Source: CAD feature listing. Evaluate the final solid. Frame: model axes, mm. Coordinates: 2 decimals unless noted, no trailing zeros. Order: outer loops, then holes, each group sorted by start corner. A loop starts at its lowest first (then second) coordinate and runs counter-clockwise, first axis right, second up.
Item 1: Contact query for flat-ended pins moving along their axis: P1, Ø3.5, axis at x = 100, z = 130, coming from the +Y side; P2, Ø8, axis at x = -108, z = 30.32, coming from the -Y side. Output: stop coordinate, or through.
Item 2: Section B-B on z = -89.5. Return the cut outline in (x, y), then the cut area to 3 significant figures.
Item 3: Section C-C on z = -40.5. Return the cut outline in (x, y), then the cut area to 3 significant figures.
Item 4: Mould query, pull axis X, two halves, no side actions, for faces 1 (the flat face through (130, 3, 2)), 2 (the flat face through (-100, 3, 78)). Classes: released by +X, released by -X, zero draft, split by the parting line, or undercut.
Item 5: Ray query, line 1 (X direction, y = 4.75, z = 130); line 2 (Z direction, x = 39.5, y = 1); line 3 (Z direction, x = -108, y = 2.75). Return the intervals inside material, ascending.
Item 6: Section D-D on y = 1.5. State how many separate pieces and enclosed holes the cut face has, then the cut area to 3 significant figures.
Item 7: Section A-A on z = -124.5. Return the cut outline in (x, y), then the cut area to 3 significant figures.
from build123d import *

# Parameters (mm, degrees)
SKETCH1_W                           = 240
SKETCH1_H                           = 320
BOSS_EXTRUDE1_DEPTH                 = 6.35
F_7_1_7_1_DIAMETER_HOLE1_D          = 7.1
M5X0_8_TAPPED_HOLE1_D               = 4.2
M5X0_8_TAPPED_HOLE3_D               = 4.2
F_5_0MM_CLEARANCE_DOWEL_SLOT1_DEPTH = 6.35
SKETCH12_W                          = 25
SKETCH12_H                          = 20
SKETCH12_W_2                        = 90
SKETCH12_H_2                        = 64.68
SKETCH12_W_3                        = 56.4
SKETCH12_H_3                        = 69.68
SKETCH12_W_4                        = 23.6
SKETCH12_H_4                        = 15
SKETCH12_H_5                        = 30.64
CUT_EXTRUDE1_DEPTH                  = 10
FILLET1_R                           = 4
FILLET1_OF_MIRROR1_R                = 4
SKETCH13_W                          = 10
SKETCH13_H                          = 320
BOSS_EXTRUDE2_DEPTH                 = 6.35
M3X0_5_TAPPED_HOLE1_D               = 2.5


# Read off the part's stored shape, not the designer's step: Ø5.0mm Clearance Dowel Slot1
with BuildPart() as part:
    # Sketch1 → Boss-Extrude1 (new body)
    with BuildSketch(Plane(origin=(0, 0, 0), x_dir=(1, 0, 0), z_dir=(0, 1, 0))):
        Rectangle(SKETCH1_W, SKETCH1_H)
    extrude(amount=BOSS_EXTRUDE1_DEPTH)

    # Ø7.1 (7.1) Diameter Hole1 (through all)
    with Locations(Plane(origin=(0, 6.35, 0), x_dir=(1, 0, 0), z_dir=(0, 1, 0))):
        with Locations((-108, 30.32), (108, 30.32), (108, -30.32), (-108, -30.32)):
            Hole(F_7_1_7_1_DIAMETER_HOLE1_D / 2)

    # M5x0.8 Tapped Hole1 (through all)
    with Locations(Plane(origin=(0, 6.35, 0), x_dir=(1, 0, 0), z_dir=(0, 1, 0))):
        with Locations((-90, 30), (-30, 30), (30, 30), (90, 30), (-90, -30), (-30, -30), (30, -30), (90, -30)):
            Hole(M5X0_8_TAPPED_HOLE1_D / 2)

    # M5x0.8 Tapped Hole3 (through all)
    with Locations(Plane(origin=(0, 6.35, 0), x_dir=(1, 0, 0), z_dir=(0, 1, 0))):
        with Locations((-80, -150), (-60, -150), (-40, -130), (-100, -130), (-100, 150), (-80, 130), (-60, 130), (-40, 150), (40, 150), (60, 130), (80, 130), (100, 150), (40, -130), (100, -130), (60, -150), (80, -150)):
            Hole(M5X0_8_TAPPED_HOLE3_D / 2)

    # Ø5.0mm Clearance Dowel Slot1 outline → Ø5.0mm Clearance Dowel Slot1 (cut)
    with BuildSketch(Plane(origin=(0, 0, 0), x_dir=(1, 0, 0), z_dir=(0, 1, 0))):
        with BuildLine():
            Line((26.15, 32.23), (26.15, 47.13))
            ThreePointArc((26.15, 47.13), (23.6, 49.68), (21.05, 47.13))
            Line((21.05, 47.13), (21.05, 32.23))
            ThreePointArc((21.05, 32.23), (23.6, 29.68), (26.15, 32.23))
        make_face()
        with BuildLine():
            ThreePointArc((26.15, 94.33), (23.6, 96.88), (21.05, 94.33))
            Line((21.05, 94.33), (21.05, 79.43))
            ThreePointArc((21.05, 79.43), (23.6, 76.88), (26.15, 79.43))
            Line((26.15, 79.43), (26.15, 94.33))
        make_face()
        with BuildLine():
            Line((-21.05, 32.23), (-21.05, 47.13))
            ThreePointArc((-21.05, 47.13), (-23.6, 49.68), (-26.15, 47.13))
            Line((-26.15, 47.13), (-26.15, 32.23))
            ThreePointArc((-26.15, 32.23), (-23.6, 29.68), (-21.05, 32.23))
        make_face()
        with BuildLine():
            ThreePointArc((-21.05, 94.33), (-23.6, 96.88), (-26.15, 94.33))
            Line((-26.15, 94.33), (-26.15, 79.43))
            ThreePointArc((-26.15, 79.43), (-23.6, 76.88), (-21.05, 79.43))
            Line((-21.05, 79.43), (-21.05, 94.33))
        make_face()
    extrude(amount=F_5_0MM_CLEARANCE_DOWEL_SLOT1_DEPTH, mode=Mode.SUBTRACT)

    # Sketch12 → Cut-Extrude1 (cut)
    with BuildSketch(Plane(origin=(0, 6.35, 0), x_dir=(1, 0, 0), z_dir=(0, 1, 0))):
        with Locations((-12.5, -135)):
            Rectangle(SKETCH12_W, SKETCH12_H)
        with Locations((-55, -77.66)):
            Rectangle(SKETCH12_W_2, SKETCH12_H_2)
        with Locations((-71.8, 80.16)):
            Rectangle(SKETCH12_W_3, SKETCH12_H_3)
        with Locations((-11.8, 122.5)):
            Rectangle(SKETCH12_W_4, SKETCH12_H_4)
        Polygon((0, 130), (-23.6, 130), (-8.6, 145), (0, 145), align=None)
        with Locations((-55, 0)):
            Rectangle(SKETCH12_W_2, SKETCH12_H_5)
    cut_extrude1 = extrude(amount=-CUT_EXTRUDE1_DEPTH, mode=Mode.SUBTRACT)

    # Fillet1
    fillet1_edges = [part.edges().sort_by_distance(p)[0] for p in [
        (-25, 3.175, 125),
        (-25, 3.175, 145),
        (-10, 3.175, 45.32),
        (-10, 3.175, 110),
        (-100, 3.175, 110),
        (-100, 3.175, 45.32),
        (-43.6, 3.175, -115),
        (-43.6, 3.175, -45.32),
        (-100, 3.175, -45.32),
        (-100, 3.175, -115),
        (-23.6, 3.175, -115),
        (-23.6, 3.175, -130),
        (-8.6, 3.175, -145),
        (-100, 3.175, 15.32),
        (-100, 3.175, -15.32),
        (-10, 3.175, -15.32),
        (-10, 3.175, 15.32),
    ]]
    fillet(fillet1_edges, radius=FILLET1_R)

    # Mirror1: Cut-Extrude1 across plane
    add(cut_extrude1.mirror(Plane.ZY), mode=Mode.SUBTRACT)

    # Fillet1 of Mirror1
    fillet1_of_mirror1_edges = [part.edges().sort_by_distance(p)[0] for p in [
        (25, 3.175, 125),
        (25, 3.175, 145),
        (10, 3.175, 45.32),
        (10, 3.175, 110),
        (100, 3.175, 110),
        (100, 3.175, 45.32),
        (43.6, 3.175, -115),
        (43.6, 3.175, -45.32),
        (100, 3.175, -45.32),
        (100, 3.175, -115),
        (23.6, 3.175, -115),
        (23.6, 3.175, -130),
        (8.6, 3.175, -145),
        (100, 3.175, 15.32),
        (100, 3.175, -15.32),
        (10, 3.175, -15.32),
        (10, 3.175, 15.32),
    ]]
    fillet(fillet1_of_mirror1_edges, radius=FILLET1_OF_MIRROR1_R)

    # Sketch13 → Boss-Extrude2 (add)
    with BuildSketch(Plane(origin=(0, 6.35, 0), x_dir=(1, 0, 0), z_dir=(0, 1, 0))):
        with Locations((-125, 0)):
            Rectangle(SKETCH13_W, SKETCH13_H)
        with Locations((125, 0)):
            Rectangle(SKETCH13_W, SKETCH13_H)
    extrude(amount=-BOSS_EXTRUDE2_DEPTH)

    # M3x0.5 Tapped Hole1 (through all)
    with Locations(Plane(origin=(0, 0, 0), x_dir=(-1, 0, 0), z_dir=(0, -1, 0))):
        with Locations((-115, 154), (115, 154)):
            Hole(M3X0_5_TAPPED_HOLE1_D / 2)


solid = part.part
Answer list:
1. P1: passes through
1. P2: stops at y = 0
2. outline: (-130, 0) - (-100, 0) - (-100, 6.35) - (-130, 6.35) - close; (-43.6, 0) - (-26.15, 0) - (-26.15, 6.35) - (-43.6, 6.35) - close; (-21.05, 0) - (21.05, 0) - (21.05, 6.35) - (-21.05, 6.35) - close; (26.15, 0) - (43.6, 0) - (43.6, 6.35) - (26.15, 6.35) - close; (100, 0) - (130, 0) - (130, 6.35) - (100, 6.35) - close
2. area: 870 mm2
3. outline: (-130, 0) - (-26.15, 0) - (-26.15, 6.35) - (-130, 6.35) - close; (-21.05, 0) - (21.05, 0) - (21.05, 6.35) - (-21.05, 6.35) - close; (26.15, 0) - (130, 0) - (130, 6.35) - (26.15, 6.35) - close
3. area: 1,590 mm2
4. face 1: released by +X
4. face 2: undercut
5. line 1: x = -130 to -102.1, -97.9 to -42.1, -37.9 to -25, 25 to 37.9, 42.1 to 97.9, 102.1 to 130
5. line 2: z = -160 to -152.04, -147.96 to -15.32, 15.32 to 45.32, 110 to 127.96, 132.04 to 160
5. line 3: z = -160 to -33.87, -26.77 to 26.77, 33.87 to 160
6. separate pieces: 1
6. enclosed holes: 42
6. area: 55,200 mm2
7. outline: (-130, 0) - (-23.6, 0) - (-23.6, 6.35) - (-130, 6.35) - close; (23.6, 0) - (130, 0) - (130, 6.35) - (23.6, 6.35) - close
7. area: 1,350 mm2
